Autodesk Fusion 360 part; units mm, degrees
sketch "Sketch1" plane through (0, 0, 0) normal (0, 0, 1) x (1, 0, 0)
  circle A0 centre (0, 0) radius 9.35
  circle A1 centre (25, 0) radius 9.35
  circle A2 centre (0, 25) radius 9.35
  circle A3 centre (25, 25) radius 9.35
  line L0 (-15, -15) -> (40, -15)
  line L1 (40, -15) -> (40, 40)
  line L2 (40, 40) -> (-15, 40)
  line L3 (-15, 40) -> (-15, -15)
  dimension "d1" = 18.7
  dimension "d4" = 25
  dimension "d5" = 25
extrude "Extrude1" add sketch "Sketch1" along normal blind 10
fillet "Fillet1" radius 2 4 edges at (-15, -15, 5) (-15, 40, 5) (40, -15, 5) (40, 40, 5)
sketch "Sketch2" plane through (0, 0, 0) normal (0, 0, -1) x (1, 0, 0)
  circle A0 centre (25, 0) radius 9.35
  circle A1 centre (0, 0) radius 9.35
  circle A2 centre (25, -25) radius 9.35
  circle A3 centre (0, -25) radius 9.35
  arc A4 (38, -40) -> (40, -38) centre (38, -38) ccw
  line L0 (40, -38) -> (40, 13)
  arc A5 (40, 13) -> (38, 15) centre (38, 13) ccw
  line L1 (38, 15) -> (-13, 15)
  arc A6 (-13, 15) -> (-15, 13) centre (-13, 13) ccw
  line L2 (-15, 13) -> (-15, -38)
  arc A7 (-15, -38) -> (-13, -40) centre (-13, -38) ccw
  line L3 (-13, -40) -> (38, -40)
  line L4 (-5, -5) -> (5, -5)
  line L5 (5, -5) -> (5, -20)
  line L6 (5, -20) -> (-5, -20)
  line L7 (-5, -20) -> (-5, -5)
  line L8 (5, -5) -> (20, -5)
  line L9 (20, -5) -> (20, 5)
  line L10 (20, 5) -> (5, 5)
  line L11 (5, 5) -> (5, -5)
  line L12 (20, -5) -> (30, -5)
  line L13 (30, -5) -> (30, -20)
  line L14 (30, -20) -> (20, -20)
  line L15 (20, -20) -> (20, -5)
  line L16 (5, -20) -> (20, -20)
  line L17 (20, -20) -> (20, -30)
  line L18 (20, -30) -> (5, -30)
  line L19 (5, -30) -> (5, -20)
  line L20 (-20, 5) -> (-5, 5)
  line L21 (-5, 5) -> (-5, -5)
  line L22 (-5, -5) -> (-20, -5)
  line L23 (-20, -5) -> (-20, 5)
  line L24 (30, -20) -> (45, -20)
  line L25 (45, -20) -> (45, -30)
  line L26 (45, -30) -> (30, -30)
  line L27 (30, -30) -> (30, -20)
extrude "Extrude2" cut sketch "Sketch2" against normal blind 3 contours A0 A1 L8 L10 | A0 A2 L13 L15 | A1 L2 L20 L22 | A2 L0 L24 L26 | A1 A3 L5 L7 | A2 A3 L16 L18
Geometry check sheet. Reference: the model listing, model coordinates, mm. A direction names the side the tool comes from. Give positions to 0.01 mm unless a question says otherwise; leave off trailing zeros. Write each loop counter-clockwise with the first axis right and the second up, starting at its lowest first coordinate (ties: lowest second). Pieces come first, ordered by that corner, then holes.
1) Material ranges on L1, parallel to X at y = 25, z = 8.25; L2, parallel to Y at x = 0, z = 2, recorded low to high.
2) Section check C-C, the plane x = 25. Record the boundary of the cut face in (y, z), and give its area (3 significant figures).
3) Section check D-D, the plane z = 5.5. Record the boundary of the cut face in (x, y).
4) Access from +Z, -Z, +X, -X, +Y, -Y to the whole of each face (thin tool, end or side, straight path). Record for faces 1 (the flat face through (36, 20, 1)), 2 (the flat face through (20, 13, 1)), 3 (the flat face through (12, 0, 3)).
5) Gauge pin test, flat ends, axial feed: pin 1 (17 mm diameter, centred on x = 25, y = 0, fed in from -Z); pin 2 (3 mm diameter, centred on x = -1, y = 11, fed in from -Z). Record the tip position at first contact, or that the pin passes through.
6) Release check for a two-part mould opening along Y. For faces 4 (the flat face through (40, 12, 5)), 5 (the flat face through (-12, -5, 1)), 6 (the flat face through (12, -15, 5)), 7 (the cylindrical face through (39.43, 39.4, 5.07)) record: pulls with the +Y half, pulls with the -Y half, needs draft (parallel to the pull), parting line crosses it, or undercut.
7) Section check A-A, the plane y = 0. Record the boundary of the cut face in (x, z), and give its area (3 significant figures).
8) Section check B-B, the plane z = 1. State how many separate pieces and enclosed holes the cut face has, and give its area (3 significant figures).
Computed:
1. L1: x = -15 to -9.35, 9.35 to 15.65, 34.35 to 40
1. L2: y = -15 to -9.35, 34.35 to 40
2. outline: (-15, 0) - (-9.35, 0) - (-9.35, 10) - (-15, 10) - close; (9.35, 3) - (15.65, 3) - (15.65, 10) - (9.35, 10) - close; (34.35, 0) - (40, 0) - (40, 10) - (34.35, 10) - close
2. area: 157 mm2
3. outline: (-15, -13) arc R2 ccw to (-13, -15) - (38, -15) arc R2 ccw to (40, -13) - (40, 38) arc R2 ccw to (38, 40) - (-13, 40) arc R2 ccw to (-15, 38) - close; hole circle Ø18.7 at (0, 0); hole circle Ø18.7 at (0, 25); hole circle Ø18.7 at (25, 0); hole circle Ø18.7 at (25, 25)
4. face 1: -Z, +X
4. face 2: -Z
4. face 3: -Z, -X
5. pin 1: passes through
5. pin 2: stops at z = 3
6. face 4: needs draft
6. face 5: undercut
6. face 6: pulls with the -Y half
6. face 7: pulls with the +Y half
7. outline: (-15, 3) - (-9.35, 3) - (-9.35, 10) - (-15, 10) - close; (9.35, 3) - (15.65, 3) - (15.65, 10) - (9.35, 10) - close; (34.35, 0) - (40, 0) - (40, 10) - (34.35, 10) - close
7. area: 140 mm2
8. separate pieces: 3
8. enclosed holes: 0
8. area: 1,510 mm2
